```python
from build123d import *

# Parameters (mm, degrees)
SKETCH1_W           = 381
SKETCH1_H           = 25.4
BOSS_EXTRUDE1_DEPTH = 50.8
SKETCH2_W           = 19.05
SKETCH2_H           = 44.45
CUT_EXTRUDE1_DEPTH  = 386.210072558
SKETCH3_R           = 3.175
CUT_EXTRUDE2_DEPTH  = 386.210072558
CUT_EXTRUDE3_START  = -25.4
CUT_EXTRUDE3_DEPTH  = 25.4
SKETCH7_R           = 2.75
CUT_EXTRUDE4_DEPTH  = 386.210072558
CUT_EXTRUDE5_REACH  = 387.21
SKETCH8_R           = 6
SKETCH8_R_2         = 1.05


with BuildPart() as part:
    # Sketch1 → Boss-Extrude1 (new body)
    with BuildSketch(Plane(origin=(0, 0, 0), x_dir=(1, 0, 0), z_dir=(0, 1, 0))):
        with Locations((-190.5, 12.7)):
            Rectangle(SKETCH1_W, SKETCH1_H)
    extrude(amount=BOSS_EXTRUDE1_DEPTH)

    # Sketch2 → Cut-Extrude1 (cut, through all)
    with BuildSketch(Plane.ZY.offset(381)):
        with Locations((-12.7, 25.4)):
            Rectangle(SKETCH2_W, SKETCH2_H)
    extrude(amount=-CUT_EXTRUDE1_DEPTH, mode=Mode.SUBTRACT)

    # Sketch3 → Cut-Extrude2 (cut, through all)
    with BuildSketch(Plane(origin=(0, 0, -25.4), x_dir=(-1, 0, 0), z_dir=(0, 0, -1))):
        with Locations((351, 26.848062316)):
            Circle(SKETCH3_R)
        with Locations(Location((30, 26.848062316, 0), (0, 0, 270))):
            Circle(SKETCH3_R)
    extrude(amount=-CUT_EXTRUDE2_DEPTH, mode=Mode.SUBTRACT)

    # Sketch5 → Cut-Extrude3 (cut)
    with BuildSketch(Plane.XY.offset(CUT_EXTRUDE3_START)):
        Polygon((-75, 32.9), (-75, 40.4), (-140, 40.4), (-140, 10.4), (-75, 10.4), (-75, 17.9), (-55, 17.9), (-55, 32.9), align=None)
    extrude(amount=CUT_EXTRUDE3_DEPTH, mode=Mode.SUBTRACT)

    # Sketch7 → Cut-Extrude4 (cut, through all)
    with BuildSketch(Plane.XY):
        with Locations((-145, 33.982591354)):
            Circle(SKETCH7_R)
        with Locations((-70, 33.982591354)):
            Circle(SKETCH7_R)
        with Locations((-145, 16.982591354)):
            Circle(SKETCH7_R)
        with Locations((-70, 16.982591354)):
            Circle(SKETCH7_R)
    extrude(amount=-CUT_EXTRUDE4_DEPTH, mode=Mode.SUBTRACT)

    # Sketch8 → Cut-Extrude5 (cut, up to next)
    with BuildSketch(Plane.XY, mode=Mode.PRIVATE) as cut_extrude5_sk1:
        with Locations((-30, 26.848062316)):
            Circle(SKETCH8_R)
    cut_extrude5_tool1 = extrude(cut_extrude5_sk1.sketch, amount=-CUT_EXTRUDE5_REACH, mode=Mode.PRIVATE) & part.part
    # Sketch8 → Cut-Extrude5 (cut, up to next)
    with BuildSketch(Plane.XY, mode=Mode.PRIVATE) as cut_extrude5_sk2:
        with Locations((-30, 38.848062316)):
            Circle(SKETCH8_R_2)
    cut_extrude5_tool2 = extrude(cut_extrude5_sk2.sketch, amount=-CUT_EXTRUDE5_REACH, mode=Mode.PRIVATE) & part.part
    # Sketch8 → Cut-Extrude5 (cut, up to next)
    with BuildSketch(Plane.XY, mode=Mode.PRIVATE) as cut_extrude5_sk3:
        with Locations((-21.514718626, 35.33334369)):
            Circle(SKETCH8_R_2)
    cut_extrude5_tool3 = extrude(cut_extrude5_sk3.sketch, amount=-CUT_EXTRUDE5_REACH, mode=Mode.PRIVATE) & part.part
    # Sketch8 → Cut-Extrude5 (cut, up to next)
    with BuildSketch(Plane.XY, mode=Mode.PRIVATE) as cut_extrude5_sk4:
        with Locations((-18, 26.848062316)):
            Circle(SKETCH8_R_2)
    cut_extrude5_tool4 = extrude(cut_extrude5_sk4.sketch, amount=-CUT_EXTRUDE5_REACH, mode=Mode.PRIVATE) & part.part
    # Sketch8 → Cut-Extrude5 (cut, up to next)
    with BuildSketch(Plane.XY, mode=Mode.PRIVATE) as cut_extrude5_sk5:
        with Locations((-21.514718626, 18.362780942)):
            Circle(SKETCH8_R_2)
    cut_extrude5_tool5 = extrude(cut_extrude5_sk5.sketch, amount=-CUT_EXTRUDE5_REACH, mode=Mode.PRIVATE) & part.part
    # Sketch8 → Cut-Extrude5 (cut, up to next)
    with BuildSketch(Plane.XY, mode=Mode.PRIVATE) as cut_extrude5_sk6:
        with Locations((-30, 14.848062316)):
            Circle(SKETCH8_R_2)
    cut_extrude5_tool6 = extrude(cut_extrude5_sk6.sketch, amount=-CUT_EXTRUDE5_REACH, mode=Mode.PRIVATE) & part.part
    # Sketch8 → Cut-Extrude5 (cut, up to next)
    with BuildSketch(Plane.XY, mode=Mode.PRIVATE) as cut_extrude5_sk7:
        with Locations((-38.485281374, 18.362780942)):
            Circle(SKETCH8_R_2)
    cut_extrude5_tool7 = extrude(cut_extrude5_sk7.sketch, amount=-CUT_EXTRUDE5_REACH, mode=Mode.PRIVATE) & part.part
    # Sketch8 → Cut-Extrude5 (cut, up to next)
    with BuildSketch(Plane.XY, mode=Mode.PRIVATE) as cut_extrude5_sk8:
        with Locations((-42, 26.848062316)):
            Circle(SKETCH8_R_2)
    cut_extrude5_tool8 = extrude(cut_extrude5_sk8.sketch, amount=-CUT_EXTRUDE5_REACH, mode=Mode.PRIVATE) & part.part
    # Sketch8 → Cut-Extrude5 (cut, up to next)
    with BuildSketch(Plane.XY, mode=Mode.PRIVATE) as cut_extrude5_sk9:
        with Locations((-38.485281374, 35.33334369)):
            Circle(SKETCH8_R_2)
    cut_extrude5_tool9 = extrude(cut_extrude5_sk9.sketch, amount=-CUT_EXTRUDE5_REACH, mode=Mode.PRIVATE) & part.part
    add(cut_extrude5_tool1.solids().sort_by_distance((-30, 26.848062, 0))[0], mode=Mode.SUBTRACT)
    add(cut_extrude5_tool2.solids().sort_by_distance((-30, 38.848062, 0))[0], mode=Mode.SUBTRACT)
    add(cut_extrude5_tool3.solids().sort_by_distance((-21.514719, 35.333344, 0))[0], mode=Mode.SUBTRACT)
    add(cut_extrude5_tool4.solids().sort_by_distance((-18, 26.848062, 0))[0], mode=Mode.SUBTRACT)
    add(cut_extrude5_tool5.solids().sort_by_distance((-21.514719, 18.362781, 0))[0], mode=Mode.SUBTRACT)
    add(cut_extrude5_tool6.solids().sort_by_distance((-30, 14.848062, 0))[0], mode=Mode.SUBTRACT)
    add(cut_extrude5_tool7.solids().sort_by_distance((-38.485281, 18.362781, 0))[0], mode=Mode.SUBTRACT)
    add(cut_extrude5_tool8.solids().sort_by_distance((-42, 26.848062, 0))[0], mode=Mode.SUBTRACT)
    add(cut_extrude5_tool9.solids().sort_by_distance((-38.485281, 35.333344, 0))[0], mode=Mode.SUBTRACT)


solid = part.part
```
Here's how the part is built. I have some questions about the finished solid (model axes, mm). A direction names the side the tool comes from. Round coordinates to 2 decimals unless told otherwise and drop trailing zeros. Order: outer loops, then holes, each group sorted by start corner. A loop starts at its lowest first (then second) coordinate and runs counter-clockwise, first axis right, second up. Notation, with made-up numbers: (32.25, 37) -> (85.25, 37) arc R23 cw to (85.25, 53) -> close; hole circle Ø11 at (-16, 3.5). An arc over 180 degrees is marked (long way). Use a Markdown table: item, result. Add a question column.
(1) If we mould it in two halves opening along Z, with no side actions, what happens to faces 1 (the face through (-193, 25, -3.175)), 2 (the face through (-381, 27, -2)), 3 (the face through (-193, 25, 0))? For each: released by +Z, released by -Z, zero draft, split by the parting line, or undercut.
(2) Suppose I cut it at A-A, the plane x = -351. Please give me the cut outline in (y, z) (3 decimals).
(3) For pin 1 Ø8 at (y, z) = (13.5, -16) entering from -X, with a flat end and sliding along its axis, tell me the tip position at first contact or that it passes through.
(4) I need wall thicknesses on line 1 along Y through (x, z) = (-145, -2.05); line 2 along Y through (x, z) = (-262.5, -20) (3 decimals); line 3 along Z through (x, y) = (-348.5, 34.5) (3 decimals). Which ranges of each line are inside material? Lowest first, please.
(5) For faces 4 (the face through (-34.422, 30.903, -1.565)), 5 (the face through (-193, 47.625, -13)), 6 (the face through (-354.03, 27.8, -1.61)), which set-ups out of +Z, -Z, +X, -X, +Y, -Y let a thin tool reach every point of the face, with its end or its side?
(6) Suppose I cut it at B-B, the plane z = -9.25. Please give me the cut outline in (x, y) (3 decimals), and give its area (3 significant figures).
Verdict:
| question | item | result |
|---|---|---|
| 1 | face 1 | undercut |
| 1 | face 2 | zero draft |
| 1 | face 3 | released by +Z |
| 2 | outline | (0, -25.4) -> (23.673, -25.4) -> (23.673, -22.225) -> (3.175, -22.225) -> (3.175, -3.175) -> (23.673, -3.175) -> (23.673, 0) -> (0, 0) -> close; (30.023, -25.4) -> (50.8, -25.4) -> (50.8, 0) -> (30.023, 0) -> (30.023, -3.175) -> (47.625, -3.175) -> (47.625, -22.225) -> (30.023, -22.225) -> close |
| 3 | pin 1 | through |
| 4 | line 1 | 0 to 14.23, 19.73 to 31.23, 36.73 to 50.8 |
| 4 | line 2 | 0 to 3.175, 47.625 to 50.8 |
| 4 | line 3 | -25.4 to -22.225, -3.175 to 0 |
| 5 | face 4 | +Z |
| 5 | face 5 | +X, -X |
| 5 | face 6 | +Z, -Z |
| 6 | outline | (-381, 0) -> (0, 0) -> (0, 3.175) -> (-381, 3.175) -> close; (-381, 47.625) -> (0, 47.625) -> (0, 50.8) -> (-381, 50.8) -> close |
| 6 | area | 2,420 mm2 |
